from build123d import *

# Parameters (mm, degrees)
F0_W     = 50
F0_H     = 60
F0_R     = 19.5
F1_DEPTH = 25
F2_R     = 15
F3_R     = 15
F4_R     = 19.5
F5_DEPTH = 5


with BuildPart() as f1:
    # F0 (on Top) → F1 (new body)
    with BuildSketch(Plane.XY):
        Rectangle(F0_W, F0_H)
        with Locations((0, 5.5)):
            Circle(F0_R, mode=Mode.SUBTRACT)
    extrude(amount=F1_DEPTH)

    # F2
    f2_edges = [f1.edges().sort_by_distance(p)[0] for p in [
        (-25, 30, 12.5),
    ]]
    fillet(f2_edges, radius=F2_R)

    # F3
    f3_edges = [f1.edges().sort_by_distance(p)[0] for p in [
        (25, 30, 12.5),
    ]]
    fillet(f3_edges, radius=F3_R)

    # F4 (on face) → F5 (join)
    with BuildSketch(Plane(origin=(0, 0, 0), x_dir=(1, 0, 0), z_dir=(0, 0, -1))):
        with Locations((0, -5.5)):
            Circle(F4_R)
    extrude(amount=-F5_DEPTH)


solid = f1.part
Geometry check sheet. Reference: the model listing, model coordinates, mm. A direction names the side the tool comes from. Coordinates: 2 decimals unless noted, no trailing zeros. Loops run counter-clockwise (first coordinate to the right, second up) from the corner with the lowest first, then second, coordinate; pieces in that order, holes last. Notation, with made-up numbers: (-28, 30) - (-10, 30) arc R29 ccw to (-10, 56) - close; hole circle Ø11 at (19.25, -19.75). An arc over 180 degrees is marked (long way). Use one line per item in the form item = value. Start each with the question number.
Item 1: Thickness scan on probe 1 along X at (y, z) = (5.5, 20.5); probe 2 along Y at (x, z) = (0, 11.75); probe 3 along Z at (x, y) = (2.5, 17). Record the ranges inside material, lowest first.
Item 2: Section check B-B, the plane y = 5.5. Enter the section's corners in (x, z), and give its area (3 significant figures).
Item 3: Section check A-A, the plane z = 21. Enter the section's corners in (x, y), and give its area (3 significant figures).
Item 4: Mould release check, pull along X, two halves, no side actions. Record for faces 3 (the face through (0, -30, 12)), 4 (the face through (9, -11.8, 14.9)), 5 (the face through (-20.72, 25.49, 12.68)): +X half, -X half, draft (parallel to the pull), parting line (faces both ways), or undercut.
Item 5: Tool access check on faces 1 (the face through (0, 5, 5)), 2 (the face through (25, -8, 12)). Record the directions out of +Z, -Z, +X, -X, +Y, -Y that give a thin tool (end or side, any length) a straight path to the whole face; none if there is none.
Item 6: Section check C-C, the plane x = 0. Enter the section's corners in (y, z), and give its area (3 significant figures).
Item 7: Gauge pin test, flat ends, axial feed: pin 1 (12 mm diameter, centred on y = 23.5, z = 3, fed in from +X); pin 2 (1 mm diameter, centred on x = 13, y = 3.5, fed in from +Z); pin 3 (12 mm diameter, centred on x = 17, z = 11.5, fed in from +Y). Record the tip position at first contact, or that the pin passes through.
Computed:
q1.probe_1 = -25 to -19.5, 19.5 to 25
q1.probe_2 = -30 to -14, 25 to 30
q1.probe_3 = 0 to 5
q2.outline = (-25, 0) - (25, 0) - (25, 25) - (19.5, 25) - (19.5, 5) - (-19.5, 5) - (-19.5, 25) - (-25, 25) - close
q2.area = 470 mm2
q3.outline = (-25, -30) - (25, -30) - (25, 15) arc R15 ccw to (10, 30) - (-10, 30) arc R15 ccw to (-25, 15) - close; hole circle Ø39 at (0, 5.5)
q3.area = 1,710 mm2
q4.face_3 = draft
q4.face_4 = undercut
q4.face_5 = -X half
q5.face_1 = +Z
q5.face_2 = +Z, -Z, +X, +Y, -Y
q6.outline = (-30, 0) - (30, 0) - (30, 25) - (25, 25) - (25, 5) - (-14, 5) - (-14, 25) - (-30, 25) - close
q6.area = 720 mm2
q7.pin_1 = 24.79
q7.pin_2 = 5
q7.pin_3 = 29.97
